from build123d import *

# Parameters (mm, degrees)
F0_W     = 50
F0_H     = 40
F1_DEPTH = 10
F2_R     = 13.825
F3_DEPTH = 9
F4_R     = 13.5
F5_DEPTH = 1
F6_W     = 4.25
F6_H     = 8
F7_DEPTH = 17.515289916
F8_R     = 5.08


with BuildPart() as f1:
    # F0 (on Top) → F1 (new body)
    with BuildSketch(Plane.XY):
        Rectangle(F0_W, F0_H)
    extrude(amount=F1_DEPTH)

    # F2 (on face) → F3 (cut)
    with BuildSketch(Plane(origin=(0, 0, 0), x_dir=(1, 0, 0), z_dir=(0, 0, -1))):
        with Locations((6.175, 0)):
            Circle(F2_R)
    extrude(amount=-F3_DEPTH, mode=Mode.SUBTRACT)

    # F4 (on face) → F5 (cut, through all)
    with BuildSketch(Plane.XY.offset(10)):
        with Locations((6.175, 0)):
            Circle(F4_R)
    extrude(amount=-F5_DEPTH, mode=Mode.SUBTRACT)

    # F6 (on face) → F7 (cut, through all)
    with BuildSketch(Plane(origin=(-25, 0, 0), x_dir=(0, -1, 0), z_dir=(-1, 0, 0))):
        with Locations((0, 4)):
            Rectangle(F6_W, F6_H)
    extrude(amount=-F7_DEPTH, mode=Mode.SUBTRACT)

    # F8
    f8_edges = [f1.edges().sort_by_distance(p)[0] for p in [
        (25, -20, 5),
        (-25, -20, 5),
        (-25, 20, 5),
        (25, 20, 5),
    ]]
    fillet(f8_edges, radius=F8_R)


solid = f1.part
Read the model definition and answer for the solid it produces. Units are mm, in the model's axes. A direction names the side the tool comes from. Coordinates: 2 decimals unless noted, no trailing zeros. Loops run counter-clockwise (first coordinate to the right, second up) from the corner with the lowest first, then second, coordinate; pieces in that order, holes last. Notation, with made-up numbers: (57, -23) -> (77, -23) arc R19 ccw to (77, 0) -> close; hole circle Ø1 at (16.5, 38.5). An arc over 180 degrees is marked (long way). Answer in a Markdown table with one row per item.
Item 1: For faces 1 (the cylindrical face through (19.362, -4.153, 4.437)), 2 (the flat face through (-16, 2.125, 4)), 3 (the cylindrical face through (23.472, 18.551, 5.07)), determine the directions among +Z, -Z, +X, -X, +Y, -Y from which every point of the face is accessible in a straight line to the end or side of a thin tool.
Returned:
| item | result |
|---|---|
| face 1 | -Z |
| face 2 | -Z, -X |
| face 3 | +Z, -Z, +X, +Y |
Item 2: Straight lines are drawn through the part: line 1 along Y through (x, z) = (-16, 7.5) (3 decimals); line 2 along X through (y, z) = (0, 5.25); line 3 along Y through (x, z) = (-0.5, 4). For each, find the intervals that lie inside material, in ascending order. Write a range as [from, to].
Returned:
| item | result |
|---|---|
| line 1 | y = [-20, -2.125], [2.125, 20] |
| line 2 | x = [20, 25] |
| line 3 | y = [-20, -12.11], [12.11, 20] |
Item 3: A cutting plane is placed at D-D on z = 5.5. Determine the outline of the cut face in (x, y) (3 decimals).
Returned:
| item | result |
|---|---|
| outline | (-25, -14.92) arc R5.08 ccw to (-19.92, -20) -> (19.92, -20) arc R5.08 ccw to (25, -14.92) -> (25, 14.92) arc R5.08 ccw to (19.92, 20) -> (-19.92, 20) arc R5.08 ccw to (-25, 14.92) -> (-25, 2.125) -> (-7.486, 2.125) arc R13.825 cw (long way) to (-7.486, -2.125) -> (-25, -2.125) -> close |
Item 4: This flat-tipped pin is pushed along its axis until it touches: P1, Ø2, axis at x = -12.5, y = 0, coming from the -Z side. Where does it stop, or does it pass through?
Returned:
| item | result |
|---|---|
| P1 | stops at z = 8 |
Item 5: For a pull along X with two mould halves and no side action, classify faces 4 (the flat face through (-25, -0.2, 8.3)), 5 (the flat face through (-16, 0, 8)), 6 (the cylindrical face through (-4.54, -8.21, 9.51)) as released by +X, released by -X, zero draft, split by the parting line, or undercut.
Returned:
| item | result |
|---|---|
| face 4 | released by -X |
| face 5 | zero draft |
| face 6 | undercut |
Item 6: A cutting plane is placed at A-A on y = 0. Determine the outline of the cut face in (x, z) (3 decimals), plus the area to 4 significant figures.
Returned:
| item | result |
|---|---|
| outline | (-25, 8) -> (-7.65, 8) -> (-7.65, 9) -> (-7.325, 9) -> (-7.325, 10) -> (-25, 10) -> close; (19.675, 9) -> (20, 9) -> (20, 0) -> (25, 0) -> (25, 10) -> (19.675, 10) -> close |
| area | 85.35 mm^2 |
Item 7: A cutting plane is placed at B-B on x = -13. Determine the outline of the cut face in (y, z) (3 decimals), plus the area to 3 significant figures.
Returned:
| item | result |
|---|---|
| outline | (-20, 0) -> (-2.125, 0) -> (-2.125, 8) -> (2.125, 8) -> (2.125, 0) -> (20, 0) -> (20, 10) -> (-20, 10) -> close |
| area | 366 mm^2 |
Item 8: A cutting plane is placed at C-C on x = -1. Determine the outline of the cut face in (y, z).
Returned:
| item | result |
|---|---|
| outline | (-20, 0) -> (-11.82, 0) -> (-11.82, 9) -> (-11.44, 9) -> (-11.44, 10) -> (-20, 10) -> close; (11.44, 9) -> (11.82, 9) -> (11.82, 0) -> (20, 0) -> (20, 10) -> (11.44, 10) -> close |
